Read the model definition and answer for the solid it produces. Units are mm, in the model's axes. A direction names the side the tool comes from. Give positions to 0.01 mm unless a question says otherwise; leave off trailing zeros. Write each loop counter-clockwise with the first axis right and the second up, starting at its lowest first coordinate (ties: lowest second). Pieces come first, ordered by that corner, then holes.
```python
from build123d import *

# Parameters (mm, degrees)
SKETCH1_W                = 2
SKETCH1_H                = 5
BOSS_EXTRUDE1_DEPTH      = 15
BOSS_EXTRUDE1_2_DEPTH    = 15
SKETCH2_W                = 1
SKETCH2_H                = 5
BOSS_EXTRUDE2_DEPTH      = 5
CUT_EXTRUDE1_DEPTH       = 33.113081447
CUT_EXTRUDE1_DEPTH_BACK  = 33.113081447
SKETCH3_R                = 1.5
SWEEP1_START             = 9
SWEEP1_DEPTH             = 6
BOSS_EXTRUDE3_DEPTH      = 12
CUT_EXTRUDE2_DEPTH       = 5
FILLET1_R                = 2
BOSS_EXTRUDE6_START      = -6
SKETCH7_W                = 6
SKETCH7_H                = 2
BOSS_EXTRUDE6_DEPTH      = 51
BOSS_EXTRUDE7_DEPTH      = 3
BOSS_EXTRUDE7_DEPTH_BACK = 9
SKETCH8_R                = 1.5
FILLET2_R                = 2.5
BOSS_EXTRUDE10_DEPTH     = 10
LPATTERN1_COUNT          = 2
LPATTERN1_PITCH          = 15


# Read off the part's stored shape, not the designer's step: Sweep1
with BuildPart() as part:
    # Sketch1 → Boss-Extrude1 (new body)
    with BuildSketch(Plane(origin=(0, 0, 0), x_dir=(0, 0, -1), z_dir=(1, 0, 0))):
        with Locations((-12, 0)):
            Rectangle(SKETCH1_W, SKETCH1_H)
    extrude(amount=BOSS_EXTRUDE1_DEPTH)



with BuildPart() as body_2:
    # Sketch1 → Boss-Extrude1 2 (new body)
    with BuildSketch(Plane(origin=(0, 0, 0), x_dir=(0, 0, -1), z_dir=(1, 0, 0))):
        with Locations((12, 0)):
            Rectangle(SKETCH1_W, SKETCH1_H)
    extrude(amount=BOSS_EXTRUDE1_2_DEPTH)


with BuildPart() as part_1:
    add(part.part)

    add(body_2.part)  # Boss-Extrude2 merges body 2
    # Sketch2 → Boss-Extrude2 (add)
    with BuildSketch(Plane(origin=(15, 0, 0), x_dir=(0, 0, -1), z_dir=(1, 0, 0))):
        with Locations((12.5, 0)):
            Rectangle(SKETCH2_W, SKETCH2_H)
        with Locations((-12.5, 0)):
            Rectangle(SKETCH2_W, SKETCH2_H)
    extrude(amount=BOSS_EXTRUDE2_DEPTH)

    # Sketch3 → Cut-Extrude1 (cut, two sides: drawn at the far end of the back side and taken through both)
    with BuildSketch(Plane.XY.offset(-12).offset(-CUT_EXTRUDE1_DEPTH_BACK)):
        with Locations((17.5, 0)):
            Circle(SKETCH3_R)
    extrude(amount=CUT_EXTRUDE1_DEPTH + CUT_EXTRUDE1_DEPTH_BACK, mode=Mode.SUBTRACT)

    # Sweep1 outline → Sweep1 (add)
    with BuildSketch(Plane.YZ.offset(SWEEP1_START)):
        with BuildLine():
            ThreePointArc((2.5, -13), (15.5, 0), (2.5, 13))
            Line((2.5, 13), (2.5, 11))
            ThreePointArc((2.5, 11), (13.5, 0), (2.5, -11))
            Line((2.5, -11), (2.5, -13))
        make_face()
    extrude(amount=SWEEP1_DEPTH)

    # Sketch5 → Boss-Extrude3 (add)
    with BuildSketch(Plane(origin=(0, 0, 0), x_dir=(0, 0, -1), z_dir=(1, 0, 0))):
        with BuildLine():
            Line((-11, -2.5), (-13, -2.5))
            add(Edge.make_bspline(
                [(-13, -2.5), (-13, -8.980170496), (0, -8.980170496)],
                knots=[3.141592654, 3.141592654, 3.141592654, 4.71238898, 4.71238898, 4.71238898], degree=2, weights=[1, 0.707106781, 1]))
            Line((0, -8.980170496), (0, -7.009343108))
            add(Edge.make_bspline(
                [(-11, -2.5), (-11, -7.009343108), (0, -7.009343108)],
                knots=[3.141592654, 3.141592654, 3.141592654, 4.71238898, 4.71238898, 4.71238898], degree=2, weights=[1, 0.707106781, 1]))
        make_face()
    boss_extrude3 = extrude(amount=BOSS_EXTRUDE3_DEPTH)

    # Sketch6 → Cut-Extrude2 (cut)
    with BuildSketch(Plane.ZY):
        with BuildLine():
            Line((13, -2.5), (11, -2.5))
            add(Edge.make_bspline(
                [(0, -7.009343108), (11, -7.009343108), (11, -2.5)],
                knots=[4.71238898, 4.71238898, 4.71238898, 6.283185307, 6.283185307, 6.283185307], degree=2, weights=[1, 0.707106781, 1]))
            Line((0, -7.009343108), (0, -8.980170496))
            add(Edge.make_bspline(
                [(0, -8.980170496), (13, -8.980170496), (13, -2.5)],
                knots=[4.71238898, 4.71238898, 4.71238898, 6.283185307, 6.283185307, 6.283185307], degree=2, weights=[1, 0.707106781, 1]))
        make_face()
    cut_extrude2 = extrude(amount=-CUT_EXTRUDE2_DEPTH, mode=Mode.SUBTRACT)

    # Mirror2: Boss-Extrude3, Cut-Extrude2 across plane
    add(boss_extrude3.mirror(Plane(origin=(12, -8.980170496, 0), x_dir=(1, 0, 0), z_dir=(0, 0, 1))))
    add(cut_extrude2.mirror(Plane(origin=(12, -8.980170496, 0), x_dir=(1, 0, 0), z_dir=(0, 0, 1))), mode=Mode.SUBTRACT)

    # Fillet1
    fillet1_edges = [part_1.edges().sort_by_distance(p)[0] for p in [
        (0, -2.5, -12),
        (0, 2.5, -12),
        (0, 2.5, 12),
        (0, -2.5, 12),
    ]]
    fillet(fillet1_edges, radius=FILLET1_R)

    # Sketch7 → Boss-Extrude6 (add)
    with BuildSketch(Plane.ZY.offset(-9).offset(BOSS_EXTRUDE6_START)):
        with Locations((0, 12.5)):
            Rectangle(SKETCH7_W, SKETCH7_H)
    extrude(amount=BOSS_EXTRUDE6_DEPTH)

    # Sketch8 → Boss-Extrude7 (add, two sides: drawn at the far end of the back side and taken through both)
    with BuildSketch(Plane.XY.offset(3).offset(-BOSS_EXTRUDE7_DEPTH_BACK)):
        with Locations((-36, 12.5)):
            Circle(SKETCH8_R)
    extrude(amount=BOSS_EXTRUDE7_DEPTH + BOSS_EXTRUDE7_DEPTH_BACK)

    # Fillet2
    fillet2_edges = [part_1.edges().sort_by_distance(p)[0] for p in [
        (20, -2.5, -12.5),
        (20, -2.5, 12.5),
    ]]
    fillet(fillet2_edges, radius=FILLET2_R)

    # 3DSketch3 → Boss-Extrude10 (add)
    with BuildSketch(Plane(origin=(-10, 7.995255445, 9.529017137), x_dir=(0, 0, -1), z_dir=(1, 0, 0))):
        with BuildLine():
            Line((0, 0), (2, 0))
            ThreePointArc((2, 0), (9.529017137, 3.825899604), (17.058034273, 0))
            Line((17.058034273, 0), (19.058034273, 0))
            ThreePointArc((19.058034273, 0), (15.031388903, 4.029654263), (9.529017137, 5.504744555))
            ThreePointArc((9.529017137, 5.504744555), (4.026645371, 4.029654263), (0, 0))
        make_face()
    boss_extrude10 = extrude(amount=BOSS_EXTRUDE10_DEPTH)

    # LPattern1: Boss-Extrude10 ×2
    with Locations(*[(-i * LPATTERN1_PITCH, 0, 0) for i in range(1, LPATTERN1_COUNT)]):
        add(boss_extrude10)


solid = part_1.part
```
Item 1: Find the intervals of material crossed by line 1 along Y through (x, z) = (17.5, 12.3); line 2 along X through (y, z) = (0, 12.55); line 3 along Y through (x, z) = (-1.5, -1), in increasing order.
Result set:
line 1: y = -2.5 to -1.5, 1.5 to 2.5
line 2: x = 0 to 16, 19 to 20
line 3: y = 11.5 to 13.5
Item 2: Section A-A (y = 12.5) is taken. Give the number of separate pieces and of enclosed holes in the cut face, and give its area (3 significant figures).
Result set:
separate pieces: 3
enclosed holes: 0
area: 441 mm2
Item 3: Which of the six approach directions +Z, -Z, +X, -X, +Y, -Y give full straight-line access (tool end or side, diameter ignored) to faces 4 (the flat face through (5, 2.5, -12)), 5 (the cylindrical face through (-5.07, 11.213, 6.714)), 6 (the cylindrical face through (-5.07, 10.21, -5.24))?
Result set:
face 4: +Z, -Z, -X, +Y
face 5: +Z, +Y
face 6: +X, -Y
Item 4: Section C-C (y = 6.5) is taken. Write down the section's boundary in (x, z).
Result set:
outline: (9, -12.37) - (15, -12.37) - (15, -10.25) - (9, -10.25) - close; (9, 10.25) - (15, 10.25) - (15, 12.37) - (9, 12.37) - close
Item 5: Each of these flat-tipped pins is pushed along its axis until it touches: pin 1 Ø9 at (y, z) = (10, -4) entering from +X; pin 2 Ø12 at (x, y) = (11, 9) entering from -Z; pin 3 Ø4 at (x, z) = (-26, -9.5) entering from -Y; pin 4 Ø1.5 at (x, y) = (18, -0.5) entering from +Z. Where does it stop, or does it pass through?
Result set:
pin 1: stops at x = 15
pin 2: stops at z = -12.99
pin 3: stops at y = 8
pin 4: passes through
Item 6: Section B-B (x = -2) is taken. Write down the section's boundary in (y, z), and give its area (3 significant figures).
Result set:
outline: (8, -9.53) arc R11 ccw to (13.08, -3) - (13.5, -3) - (13.5, 3) - (13.08, 3) arc R11 ccw to (8, 9.53) - (8, 7.53) arc R9.32 cw to (11.5, 2.43) - (11.5, -2.43) arc R9.32 cw to (8, -7.53) - close
area: 36.0 mm2
Item 7: Determine the mould class of faces 1 (the flat face through (-25, 10, 6)), 2 (the flat face through (-13, 13.5, 0)), 3 (the cylindrical face through (12, 9.1, 8.8)) for opening direction Y: pulls with the +Y half, pulls with the -Y half, needs draft (parallel to the pull), parting line crosses it, or undercut.
Result set:
face 1: needs draft
face 2: pulls with the +Y half
face 3: undercut
